```python
from build123d import *

# Parameters (mm, degrees)
SKETCH1_R           = 2.5
BOSS_EXTRUDE1_DEPTH = 9
SKETCH2_W           = 5
SKETCH2_H           = 5
BOSS_EXTRUDE2_DEPTH = 2
SCALE1_SCALE        = 2


with BuildPart() as part:
    # Sketch1 → Boss-Extrude1 (new body)
    with BuildSketch(Plane(origin=(0, 0, 0), x_dir=(1, 0, 0), z_dir=(0, 1, 0))):
        with Locations(Location((0, 0, 0), (0, 0, 270))):
            Circle(SKETCH1_R)
    extrude(amount=BOSS_EXTRUDE1_DEPTH)

    # Sketch2 → Boss-Extrude2 (add)
    with BuildSketch(Plane(origin=(0, 9, 0), x_dir=(1, 0, 0), z_dir=(0, 1, 0))):
        Rectangle(SKETCH2_W, SKETCH2_H)
    extrude(amount=BOSS_EXTRUDE2_DEPTH)


with BuildPart() as part_1:
    # Scale1: scaled about (0, 5.712978856, 0)
    add(part.part.scale(SCALE1_SCALE).moved(Location((0, -5.712978856, 0))))


solid = part_1.part
```
Here's how the part is built. I have some questions about the finished solid (model axes, mm). A direction names the side the tool comes from. Give positions to 0.01 mm unless a question says otherwise; leave off trailing zeros. Write each loop counter-clockwise with the first axis right and the second up, starting at its lowest first coordinate (ties: lowest second). Pieces come first, ordered by that corner, then holes. Notation, with made-up numbers: M -27.5,40 L -4.5,40 A25 cw -4.5,54 Z; hole C 32,4 d8. An arc over 180 degrees is marked long. Put each result on its own line as item: value. Start each with the question number.
Item 1: If we section it at A-A, the plane x = -3: Write out the boundary of the cut face in (y, z), then the cut area to 3 significant figures.
Item 2: I need wall thicknesses on L1, parallel to Y at x = 2.25, z = -4.5; L2, parallel to Z at x = -3.5, y = 1; L3, parallel to Z at x = -2.75, y = 6.5. Which ranges of each line are inside material? Lowest first, please. Write a range as from..to.
Item 3: If we section it at B-B, the plane y = 10.25: Write out the boundary of the cut face in (x, z).
Item 4: If we section it at C-C, the plane z = 2.5: Write out the boundary of the cut face in (x, y).
Item 5: On a 3-axis mill with a long thin cutter (end or side, diameter ignored), from which of +Z, -Z, +X, -X, +Y, -Y can I reach the whole of each face in a straight line? I mean faces 1 (the flat face through (-4, 12.287, -4)), 2 (the cylindrical face through (-4.88, 3.16, -1.08)), 3 (the flat face through (-4, 12.287, 4)). Say none if no direction works.
Item 6: Will this pin go through, and if not, where does the flat tip stop? pin 1 (3 mm diameter, centred on x = -1.5, y = 6, fed in from -Z).
Values:
1. outline: M -5.71,-4 L 12.29,-4 L 12.29,-5 L 16.29,-5 L 16.29,5 L 12.29,5 L 12.29,4 L -5.71,4 Z
1. area: 184 mm²
2. L1: 12.29..16.29
2. L2: -3.57..3.57
2. L3: -4.18..4.18
3. outline: C 0,0 d10
4. outline: M -5,12.29 L -4.33,12.29 L -4.33,-5.71 L 4.33,-5.71 L 4.33,12.29 L 5,12.29 L 5,16.29 L -5,16.29 Z
5. face 1: -Z, -X, -Y
5. face 2: -Y
5. face 3: +Z, -X, -Y
6. pin 1: z = -5
